The drawing under review shows one solid part. Ordinate dimensions are in mm from its lowest x, y, z. Give positions to 0.01 mm unless a question says otherwise; leave off trailing zeros. Order: outer loops, then holes, each group sorted by start corner. A loop starts at its lowest first (then second) coordinate and runs counter-clockwise, first axis right, second up. Notation, with made-up numbers: (69.5, 14) - (75.5, 14) arc R7 ccw to (75.5, 25) - close; hole circle Ø9 at (0, 83.5). An arc over 180 degrees is marked (long way). Write item = value, one per line. Start each with the question number.
1. For P1, Ø22.5, axis at x = 176.9, y = 56.9, coming from the -Z side; P2, Ø8, axis at x = 81.5, y = 167.5, coming from the -Z side, all flat-tipped, find the tip position at first contact; note any pin that passes through.
2. We need section C-C, the plane z = 1.9. Give the boundary of the cut face in (x, y), and give its area (3 significant figures).
3. Wall thickness on probe 1 along Y at (x, z) = (176.9, 1.5); probe 2 along Y at (x, z) = (50, 2.45); probe 3 along X at (y, z) = (59.5, 1.85): over which ranges is each line inside the solid? List them lowest first.
4. We need section A-A, the plane x = 56.9. Give the boundary of the cut face in (y, z).
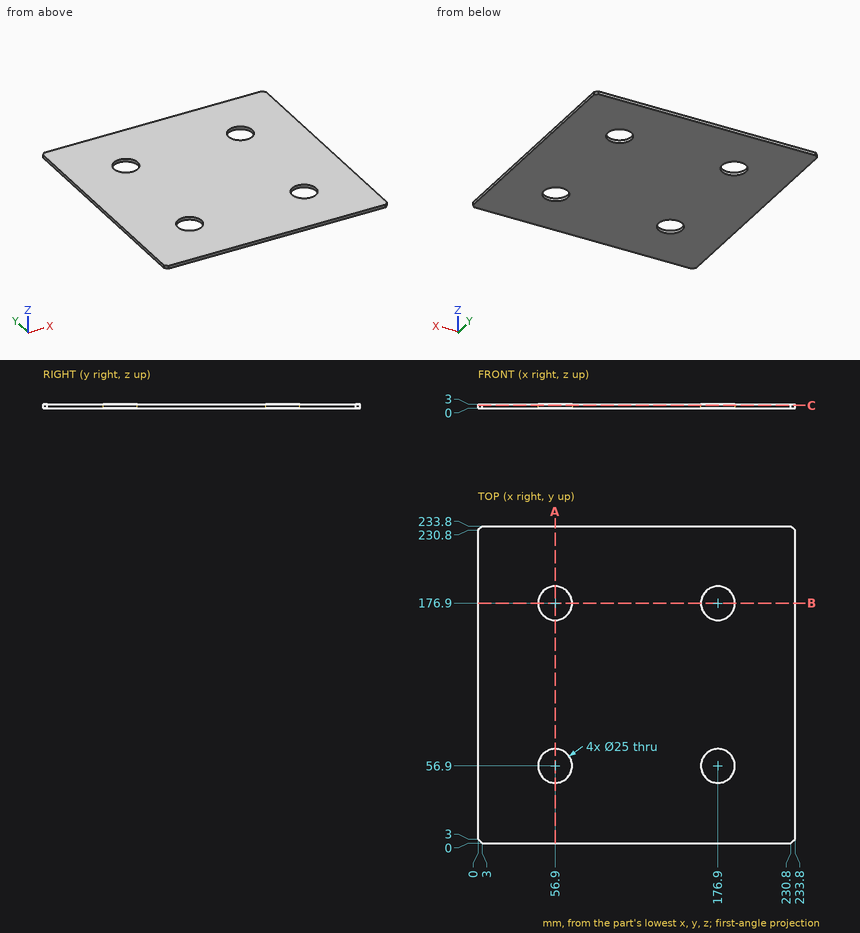
Model answer:
q1.P1 = through
q1.P2 = 0
q2.outline = (0, 3) - (3, 0) - (230.8, 0) - (233.8, 3) - (233.8, 230.8) - (230.8, 233.8) - (3, 233.8) - (0, 230.8) - close; hole circle Ø25 at (56.9, 56.9); hole circle Ø25 at (56.9, 176.9); hole circle Ø25 at (176.9, 56.9); hole circle Ø25 at (176.9, 176.9)
q2.area = 52,700 mm2
q3.probe_1 = 0 to 44.4, 69.4 to 164.4, 189.4 to 233.8
q3.probe_2 = 0 to 46.48, 67.32 to 166.48, 187.32 to 233.8
q3.probe_3 = 0 to 44.67, 69.13 to 164.67, 189.13 to 233.8
q4.outline = (0, 0) - (44.4, 0) - (44.4, 3) - (0, 3) - close; (69.4, 0) - (164.4, 0) - (164.4, 3) - (69.4, 3) - close; (189.4, 0) - (233.8, 0) - (233.8, 3) - (189.4, 3) - close
